Part model, mm, in its own coordinate system. A direction names the side the tool comes from. Coordinates: 2 decimals unless noted, no trailing zeros. Loops run counter-clockwise (first coordinate to the right, second up) from the corner with the lowest first, then second, coordinate; pieces in that order, holes last. Notation, with made-up numbers: (-33, -29) - (18, -29) arc R22 ccw to (18, -23) - close; hole circle Ø9 at (4.25, 79). An arc over 180 degrees is marked (long way). Answer as CSV lines item,"result".
Autodesk Inventor part; units mm, degrees
ref_plane "YZ Plane" through (0, 0, 0) normal (1, 0, 0) x (0, 1, 0)
ref_plane "XZ Plane" through (0, 0, 0) normal (0, 1, 0) x (-1, 0, 0)
ref_plane "XY Plane" through (0, 0, 0) normal (0, 0, 1) x (1, 0, 0)
sketch "Sketch1" plane through (0, 0, 0) normal (0, 1, 0) x (-1, 0, 0)
  line L0 (0, 0) -> (-27, 0) construction
  line L1 (-27, -8) -> (0, -8)
  arc A0 (0, -8) -> (0, 8) centre (0, 0) ccw
  arc A1 (-27, 8) -> (-27, -8) centre (-27, 0) ccw
  line L2 (14.5, 10) -> (-41.5, 10)
  line L3 (-41.5, 10) -> (-41.5, -10)
  line L4 (-41.5, -10) -> (14.5, -10)
  line L5 (14.5, -10) -> (14.5, 10)
  line L6 (14.5, 10) -> (-41.5, -10) construction
  line L7 (-41.5, 10) -> (14.5, -10) construction
  line L8 (14.5, 10) -> (-41.5, 10)
  line L9 (-41.5, 10) -> (-41.5, 15)
  line L10 (-41.5, 15) -> (14.5, 15)
  line L11 (14.5, 15) -> (14.5, 10)
  arc A2 (0, -8) -> (-5.3358, 5.9607) centre (0, 0) ccw
  arc A3 (-21.6642, 5.9607) -> (-27, -8) centre (-27, 0) ccw
  line L12 (9, -10) -> (-36, -10)
  line L13 (-36, -10) -> (-36, 10) construction
  line L14 (-36, 10) -> (9, 10)
  line L15 (9, 10) -> (9, -10) construction
  line L16 (9, -10) -> (-36, 10) construction
  line L17 (-36, -10) -> (9, 10) construction
  line L18 (9, 10) -> (-6, 10)
  line L19 (-6, 10) -> (-6, 5.9607)
  line L20 (-36, 10) -> (-21, 10)
  line L21 (-21, 10) -> (-21, 5.9607)
  line L22 (-5.3358, 5.9607) -> (-21.6642, 5.9607) construction
  line L23 (-21, 5.9607) -> (-21.6642, 5.9607)
  line L24 (-6, 5.9607) -> (-5.3358, 5.9607)
  point P0 (-13.5, 0)
  point P1 (-27, 8)
  point P2 (0, 8)
  dimension "d0" = 27
  dimension "d1" = 16
  dimension "d2" = 56
  dimension "d3" = 20
  dimension "d4" = 5
  dimension "d5" = 45
  dimension "d6" = 15
  dimension "d7" = 15
extrude "Extrusion1" add sketch "Sketch1" along normal blind 8 contours L1 A0 A2 L24 L19 L2 L5 L4 L3 L21 L23 A3 A1
extrude "Extrusion2" add sketch "Sketch1" along normal blind 15.5 contours L2 L9 L10 L11
sketch "Sketch2" plane through (21, 0, 10) normal (0, 0, -1) x (-1, 0, 0)
  line L0 (35.5, 8) -> (15, 8)
  line L1 (-20.5, 8) -> (-20.5, 15.5)
  line L2 (35.5, 8) -> (-20.5, 8)
  line L3 (-20.5, 8) -> (-20.5, 15.5)
  line L4 (-20.5, 15.5) -> (35.5, 15.5)
  line L5 (35.5, 15.5) -> (35.5, 8)
  line L6 (31, 8) -> (-16, 8)
  line L7 (-16, 8) -> (-16, 12.5)
  line L8 (-16, 12.5) -> (31, 12.5)
  line L9 (31, 12.5) -> (31, 8)
  line L10 (-20.5, 8) -> (35.5, 8)
  point P0 (21, 0)
  point P1 (7.5, 8)
  dimension "d12" = 47
  dimension "d13" = 4.5
extrude "Extrusion3" add sketch "Sketch2" along normal blind 3 contours L0 L9 L8 L7 L2 L1 L4 L5
sketch "Sketch3" plane through (41.5, 0, -10) normal (0, 0, -1) x (-1, 0, 0)
  circle A0 centre (52, 4) radius 2.15
  line L0 (56, 0) -> (56, 8)
  line L1 (0, 0) -> (56, 0)
  circle A1 centre (4, 4) radius 2.15
  line L2 (0, 0) -> (0, 8)
  point P0 (41.5, 0)
  dimension "d16" = 4.3
  dimension "d17" = 4
  dimension "d18" = 4
  dimension "d19" = 4.3
  dimension "d20" = 4
  dimension "d21" = 4
extrude "Extrusion4" cut sketch "Sketch3" against normal blind 32
properties part number "Ultrasonic_sensor_frame_Full"
Q1. Saw through at A-A (z = 0). Give the cut face in (x, y).
Results:
outline,"(-14.5, 0) - (-8, 0) - (-8, 8) - (-14.5, 8) - close; (35, 0) - (41.5, 0) - (41.5, 8) - (35, 8) - close; hole circle Ø4.3 at (-10.5, 4); hole circle Ø4.3 at (37.5, 4)"
Q2. Two-plate mould, pull along Z, no slides. Class faces 6 (the face through (14, 13, 7)), 7 (the face through (24.182, 3.944, 7.487)), 8 (the face through (13, 8, 10)), 9 (the face through (14, 0, 11)): released by +Z, released by -Z, zero draft, split by the parting line, or undercut.
Results:
face 6,"released by -Z"
face 7,"undercut"
face 8,"undercut"
face 9,"zero draft"
Q3. Saw through at C-C (x = 17.5). Give the cut face in (y, z), then the cut area to 4 significant figures.
Results:
outline,"(0, -10) - (8, -10) - (8, -8) - (0, -8) - close; (0, 10) - (12.5, 10) - (12.5, 7) - (15.5, 7) - (15.5, 15) - (0, 15) - close"
area,"102.5 mm^2"
Q4. Saw through at D-D (y = 8.75). Give the cut face in (x, z).
Results:
outline,"(-14.5, 7) - (-10, 7) - (-10, 10) - (37, 10) - (37, 7) - (41.5, 7) - (41.5, 15) - (-14.5, 15) - close"
Q5. Which spindle directions (+Z, -Z, +X, -X, +Y, -Y) get a long thin tool onto all of the face, cutting with end or side? Do faces 1 (the face through (14, 4, -10)), 2 (the face through (41.5, 6, 5)), 3 (the face through (14, 4, -8)), 4 (the face through (14, 12.5, 9)), 5 (the face through (6, 4, 8)). Say none if no direction does.
Results:
face 1,"-Z, +X, -X, +Y, -Y"
face 2,"+Z, -Z, +X, +Y, -Y"
face 3,"+Y, -Y"
face 4,"-Z"
face 5,"-Y"
Q6. Wall check: L1, parallel to Z at x = 0, y = 6.25; L2, parallel to Y at x = -10.5, z = 4.5; L3, parallel to Z at x = 29, y = 10. Give the ranges that are in metal, low to high.
Results:
L1,"z = -10 to -8, 8 to 15"
L2,"y = 0 to 1.85, 6.15 to 8"
L3,"z = 10 to 15"
Q7. Saw through at B-B (y = 4). Give the cut face in (x, z), then the cut area to 3 significant figures.
Results:
outline,"(-14.5, -10) - (-12.65, -10) - (-12.65, 15) - (-14.5, 15) - close; (-8.35, -10) - (35.35, -10) - (35.35, 15) - (-8.35, 15) - close; (39.65, -10) - (41.5, -10) - (41.5, 15) - (39.65, 15) - close; hole (0, -8) - (27, -8) arc R8 ccw to (27, 8) arc R8 ccw to (21.66, 5.96) - (21, 5.96) - (21, 10) - (6, 10) - (6, 5.96) - (5.34, 5.96) arc R8 ccw to (0, 8) arc R8 ccw to start"
area,"531 mm^2"
